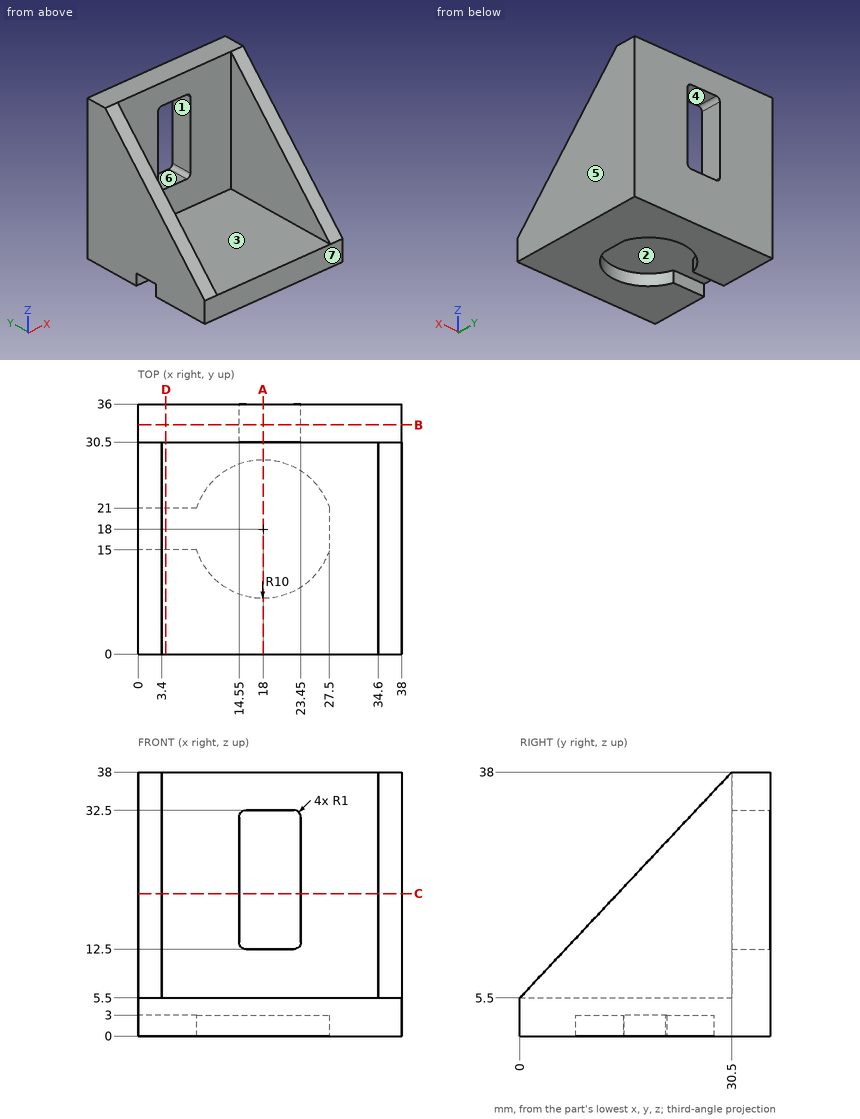
Answer from the drawing. Dimensions are ordinates in mm from the lowest x, y and z of the part. A direction names the side the tool comes from. Give positions to 0.01 mm unless a question says otherwise; leave off trailing zeros. Order: outer loops, then holes, each group sorted by start corner. A loop starts at its lowest first (then second) coordinate and runs counter-clockwise, first axis right, second up.
Item 1: The part is cut by section A-A, the plane x = 18. Give the vertices of the cut face in (y, z).
From the geometry:
outline: (0, 0) - (8, 0) - (8, 3) - (28, 3) - (28, 0) - (36, 0) - (36, 12.5) - (30.5, 12.5) - (30.5, 5.5) - (0, 5.5) - close; (30.5, 32.5) - (36, 32.5) - (36, 38) - (30.5, 38) - close
Item 2: Given pin 1 Ø2.5 at (x, z) = (6, 1) entering from -Y; pin 2 Ø1.5 at (y, z) = (18, 1.5) entering from -X; pin 3 Ø9.5 at (x, z) = (13, 24) entering from -Y; pin 4 Ø2 at (x, y) = (16.5, 25.5) entering from -Z, each flat-ended and moving along its own axis, determine where each tip first touches the part or whether it passes through.
From the geometry:
pin 1: stops at y = 0
pin 2: stops at x = 27.5
pin 3: stops at y = 30.5
pin 4: stops at z = 3
Item 3: Which of the six approach directions +Z, -Z, +X, -X, +Y, -Y give full straight-line access (tool end or side, diameter ignored) to the marked faces 1, 2 and 3?
From the geometry:
face 1: +Y, -Y
face 2: -Z
face 3: +Z, -Y
Item 4: Find the intervals of material crossed by probe 1 along X at (y, z) = (31.5, 18.5); probe 2 along X at (y, z) = (15, 18); probe 3 along Y at (x, z) = (11.5, 9), in increasing order.
From the geometry:
probe 1: x = 0 to 14.55, 23.45 to 38
probe 2: x = 0 to 3.4, 34.6 to 38
probe 3: y = 30.5 to 36
Item 5: For a pull along X with two mould halves and no side action, classify the marked faces 4, 5, 6 and 7 as pulls with the +X half, pulls with the -X half, needs draft (parallel to the pull), parting line crosses it, or undercut.
From the geometry:
face 4: undercut
face 5: pulls with the +X half
face 6: undercut
face 7: needs draft
Item 6: The part is cut by section D-D, the plane x = 4. Give the vertices of the cut face in (y, z), and give its area (3 significant figures).
From the geometry:
outline: (0, 0) - (15, 0) - (15, 3) - (21, 3) - (21, 0) - (36, 0) - (36, 38) - (30.5, 38) - (30.5, 5.5) - (0, 5.5) - close
area: 359 mm2
Item 7: The part is cut by section B-B, the plane y = 33. Give the vertices of the cut face in (x, z).
From the geometry:
outline: (0, 0) - (38, 0) - (38, 38) - (0, 38) - close; hole (14.55, 13.5) arc R1 ccw to (15.55, 12.5) - (22.45, 12.5) arc R1 ccw to (23.45, 13.5) - (23.45, 31.5) arc R1 ccw to (22.45, 32.5) - (15.55, 32.5) arc R1 ccw to (14.55, 31.5) - close
Item 8: The part is cut by section C-C, the plane z = 20.5. Give the vertices of the cut face in (x, y).
From the geometry:
outline: (0, 14.08) - (3.4, 14.08) - (3.4, 30.5) - (14.55, 30.5) - (14.55, 36) - (0, 36) - close; (23.45, 30.5) - (34.6, 30.5) - (34.6, 14.08) - (38, 14.08) - (38, 36) - (23.45, 36) - close
